The drawing under review shows one solid part. Ordinate dimensions are in mm from its lowest x, y, z. A direction names the side the tool comes from. Round coordinates to 2 decimals unless told otherwise and drop trailing zeros. Write each loop counter-clockwise with the first axis right and the second up, starting at its lowest first coordinate (ties: lowest second). Pieces come first, ordered by that corner, then holes. Notation, with made-up numbers: (66, 5.25) -> (75, 5.25) arc R32 cw to (75, 32.25) -> close; hole circle Ø10 at (14.25, 11). An arc over 180 degrees is marked (long way). Use CSV: the item, a comma, the result in double quotes. Start each with the question number.
1) Take a section at D-D, the plane y = 44. Give the boundary of the cut face in (x, z), then the cut area to 3 significant figures.
2) Take a section at A-A, the plane z = 22. Give the boundary of the cut face in (x, y), then the cut area to 3 significant figures.
3) Take a section at B-B, the plane y = 8.5. Give the boundary of the cut face in (x, z).
4) Take a section at C-C, the plane x = 39. Give the boundary of the cut face in (y, z).
5) Mouldability with a two-part tool opening along Y and no side actions: class the marked faces 6, 7 and 8 as released by +Y, released by -Y, zero draft, split by the parting line, or undercut.
6) Machinability: for the marked faces 1, 2, 3, 4 and 5, which of the approach directions +Z, -Z, +X, -X, +Y, -Y give a long, thin tool a straight path to every point of the face, cutting with its end or side? Answer none if there is none.
7) For pin 1 Ø5 at (x, y) = (58, 17) entering from +Z; pin 2 Ø5 at (x, y) = (39.5, 33.5) entering from -Z; pin 3 Ø3 at (x, z) = (28.5, 23.5) entering from +Y, all flat-tipped, find the tip position at first contact; note any pin that passes through.
8) Wall thickness on probe 1 along Y at (x, z) = (58, 32); probe 2 along Z at (x, y) = (49.5, 17): over which ranges is each line inside the solid? List them lowest first. Write a range as [from, to].
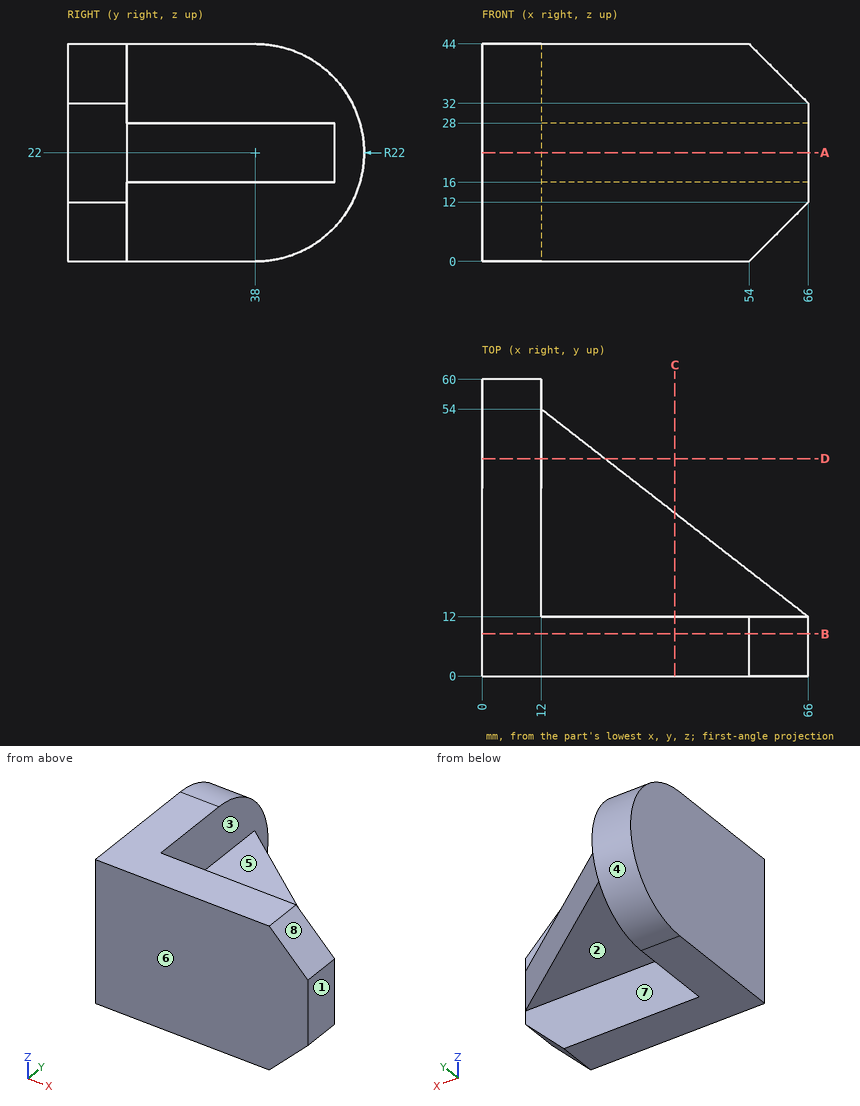
Values found:
1,outline,"(0, 0.83) -> (12, 0.83) -> (12, 16) -> (24.86, 16) -> (24.86, 28) -> (12, 28) -> (12, 43.17) -> (0, 43.17) -> close"
1,area,"662 mm²"
2,outline,"(0, 0) -> (66, 0) -> (66, 12) -> (12, 54) -> (12, 60) -> (0, 60) -> close"
2,area,"2,500 mm²"
3,outline,"(0, 0) -> (54, 0) -> (66, 12) -> (66, 32) -> (54, 44) -> (0, 44) -> close"
4,outline,"(0, 0) -> (12, 0) -> (12, 16) -> (33, 16) -> (33, 28) -> (12, 28) -> (12, 44) -> (0, 44) -> close"
5,face 6,"released by -Y"
5,face 7,"released by +Y"
5,face 8,"zero draft"
6,face 1,"+Z, -Z, +X, +Y, -Y"
6,face 2,"-Z, +X, +Y"
6,face 3,"+X, +Y"
6,face 4,"+X, -X, +Y"
6,face 5,"+Z, +X, +Y"
7,pin 1,"z = 28"
7,pin 2,"z = 16"
7,pin 3,"y = 42.33"
8,probe 1,"[0, 12]"
8,probe 2,"[16, 28]"
